Geometry check sheet. Reference: the model listing, model coordinates, mm. Face numbers are marked on the shaded views. Give positions to 0.01 mm unless a question says otherwise; leave off trailing zeros. Write each loop counter-clockwise with the first axis right and the second up, starting at its lowest first coordinate (ties: lowest second). Pieces come first, ordered by that corner, then holes. Notation, with made-up numbers: (52.25, 9) - (86.25, 9) arc R20 ccw to (86.25, 33) - close; hole circle Ø11 at (17.5, 75.5). An arc over 180 degrees is marked (long way). Use a Markdown table: item, result.
```python
from build123d import *

# Parameters (mm, degrees)
F0_R     = 50.8
F1_DEPTH = 50.8


with BuildPart() as f1:
    # F0 (on Front) → F1 (new body)
    with BuildSketch(Plane.XZ):
        Circle(F0_R)
        with BuildLine():
            ThreePointArc((-34.681557, 30.27608), (-34.29, 34.29), (-30.27608, 34.681557))
            ThreePointArc((-30.27608, 34.681557), (0, 46.0375), (30.27608, 34.681557))
            ThreePointArc((30.27608, 34.681557), (34.29, 34.29), (34.681557, 30.27608))
            ThreePointArc((34.681557, 30.27608), (46.0375, 0), (34.681557, -30.27608))
            ThreePointArc((34.681557, -30.27608), (34.29, -34.29), (30.27608, -34.681557))
            ThreePointArc((30.27608, -34.681557), (0, -46.0375), (-30.27608, -34.681557))
            ThreePointArc((-30.27608, -34.681557), (-34.29, -34.29), (-34.681557, -30.27608))
            ThreePointArc((-34.681557, -30.27608), (-46.0375, 0), (-34.681557, 30.27608))
        make_face(mode=Mode.SUBTRACT)
    extrude(amount=F1_DEPTH)


solid = f1.part
```
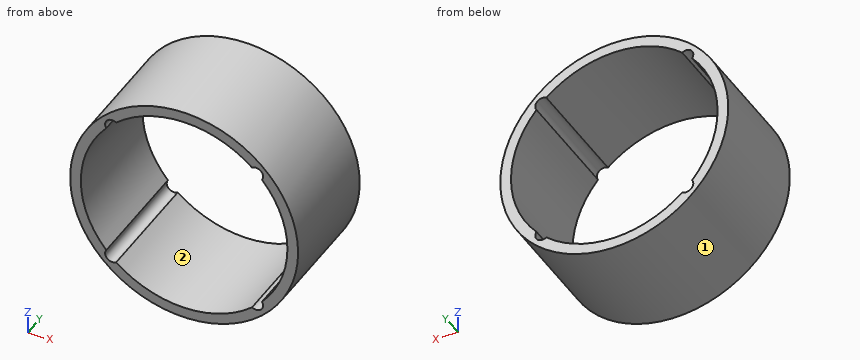
1) Section check B-B on z = 0. Record the boundary of the cut face in (x, y), then the cut area to 3 significant figures.
Working result:
| item | result |
|---|---|
| outline | (-50.8, -50.8) - (-46.04, -50.8) - (-46.04, 0) - (-50.8, 0) - close; (46.04, -50.8) - (50.8, -50.8) - (50.8, 0) - (46.04, 0) - close |
| area | 484 mm² |
2) Section check A-A on x = 0. Record the boundary of the cut face in (y, z).
Working result:
| item | result |
|---|---|
| outline | (-50.8, -50.8) - (0, -50.8) - (0, -46.04) - (-50.8, -46.04) - close; (-50.8, 46.04) - (0, 46.04) - (0, 50.8) - (-50.8, 50.8) - close |
3) Mould release check, pull along X, two halves, no side actions. Record for the marked faces 1 and 2: pulls with the +X half, pulls with the -X half, needs draft (parallel to the pull), parting line crosses it, or undercut.
Working result:
| item | result |
|---|---|
| face 1 | parting line crosses it |
| face 2 | undercut |
4) Depth check by flat-ended pin: P1, Ø12, axis at y = -33.5, z = 15, coming from the -X side; P2, Ø1.5, axis at x = -20, y = -11, coming from the -Z side; P3, Ø3, axis at y = -14.5, z = 3, coming from the +X side; P4, Ø6, axis at x = -40.5, z = -24.5, coming from the +Y side. Enter the tip coordinate at first touch or a pass-through.
Working result:
| item | result |
|---|---|
| P1 | stops at x = -50 |
| P2 | stops at z = -47.01 |
| P3 | stops at x = 50.78 |
| P4 | stops at y = 0 |
5) Material ranges on L1, parallel to X at y = -31, z = 11; L2, parallel to X at y = -32, z = 17.5; L3, parallel to Z at x = 13.5, y = -21, recorded low to high. Write a range as from..to.
Working result:
| item | result |
|---|---|
| L1 | x = -49.59..-44.7, 44.7..49.59 |
| L2 | x = -47.69..-42.58, 42.58..47.69 |
| L3 | z = -48.97..-44.01, 44.01..48.97 |
